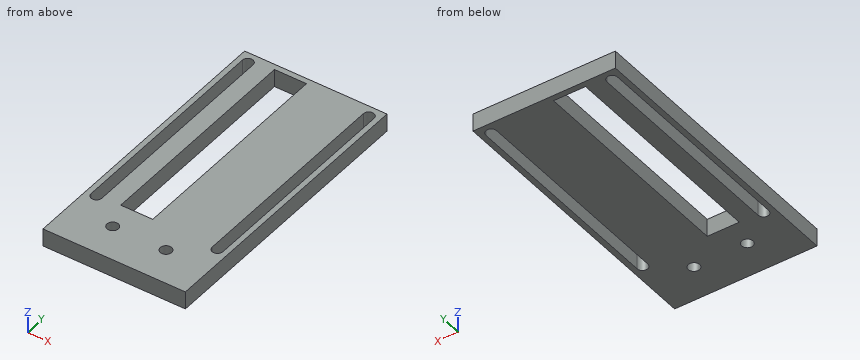
from build123d import *

# Parameters (mm, degrees)
SKETCH1_W           = 40
SKETCH1_H           = 20
SKETCH1_R           = 1.6
BOSS_EXTRUDE1_DEPTH = 5
SKETCH3_W           = 40
SKETCH3_H           = 5
BOSS_EXTRUDE3_DEPTH = 60
CUT_EXTRUDE1_DEPTH  = 73.972597597
SKETCH5_W           = 9
SKETCH5_H           = 60.997272609
CUT_EXTRUDE2_DEPTH  = 73.972597597


with BuildPart() as part:
    # Sketch1 → Boss-Extrude1 (new body)
    with BuildSketch(Plane.XY):
        Rectangle(SKETCH1_W, SKETCH1_H)
        with Locations((-7.5, 0)):
            Circle(SKETCH1_R, mode=Mode.SUBTRACT)
        with Locations((7.5, 0)):
            Circle(SKETCH1_R, mode=Mode.SUBTRACT)
    extrude(amount=BOSS_EXTRUDE1_DEPTH)

    # Sketch3 → Boss-Extrude3 (add)
    with BuildSketch(Plane(origin=(0, 10, 0), x_dir=(1, 0, 0), z_dir=(0, 1, 0))):
        with Locations((0, -2.5)):
            Rectangle(SKETCH3_W, SKETCH3_H)
    extrude(amount=BOSS_EXTRUDE3_DEPTH)

    # Sketch4 → Cut-Extrude1 (cut, through all)
    with BuildSketch(Plane(origin=(0, 0, 0), x_dir=(-1, 0, 0), z_dir=(0, 0, -1))):
        with BuildLine():
            Line((-15.5, 67), (-15.5, 7))
            ThreePointArc((-15.5, 7), (-17, 5.5), (-18.5, 7))
            Line((-18.5, 7), (-18.5, 67))
            ThreePointArc((-18.5, 67), (-17, 68.5), (-15.5, 67))
        make_face()
        with BuildLine():
            Line((18.5, 67), (18.5, 7))
            ThreePointArc((18.5, 7), (17, 5.5), (15.5, 7))
            Line((15.5, 7), (15.5, 67))
            ThreePointArc((15.5, 67), (17, 68.5), (18.5, 67))
        make_face()
    extrude(amount=-CUT_EXTRUDE1_DEPTH, mode=Mode.SUBTRACT)

    # Sketch5 → Cut-Extrude2 (cut, through all)
    with BuildSketch(Plane(origin=(0, 0, 0), x_dir=(-1, 0, 0), z_dir=(0, 0, -1))):
        with Locations((6, 37.926958335)):
            Rectangle(SKETCH5_W, SKETCH5_H)
    extrude(amount=-CUT_EXTRUDE2_DEPTH, mode=Mode.SUBTRACT)


solid = part.part
Model file for the job. Use its own axes, mm. Give positions to 0.01 mm unless a question says otherwise; leave off trailing zeros. Write each loop counter-clockwise with the first axis right and the second up, starting at its lowest first coordinate (ties: lowest second). Pieces come first, ordered by that corner, then holes. Notation, with made-up numbers: M 83,32 L 130,32 A19 cw 130,66 Z; hole C 83.5,54 d1. An arc over 180 degrees is marked long. One line per item, written item: value. Start each with the question number.
Q1. Saw through at A-A, the plane x = -7.5. Write the cut outline in (y, z), plus the area to 3 significant figures.
Q2. Probe probe 1 along X at (y, z) = (35, 1); probe 2 along Y at (x, z) = (-7.5, 3.75); probe 3 along Y at (x, z) = (7.5, 2.3). List the from-to ranges inside material, lowest first. Write a range as [from, to].
Q3. Saw through at C-C, the plane z = 0.9. Write the cut outline in (x, y), plus the area to 3 significant figures.
Q4. Saw through at D-D, the plane x = -17. Write the cut outline in (y, z), plus the area to 3 significant figures.
Q5. Drop a flat-ended pin along its axis: pin 1 Ø12 at (x, y) = (-11, 6) entering from -Z. Give the stop position or say it passes through.
Q6. Saw through at B-B, the plane y = 39.5. Write the cut outline in (x, z), plus the area to 3 significant figures.
Output values:
1. outline: M -10,0 L -1.6,0 L -1.6,5 L -10,5 Z; M 1.6,0 L 7.43,0 L 7.43,5 L 1.6,5 Z; M 68.43,0 L 70,0 L 70,5 L 68.43,5 Z
1. area: 79.0 mm²
2. probe 1: x = [-20, -18.5], [-15.5, -10.5], [-1.5, 15.5], [18.5, 20]
2. probe 2: y = [-10, -1.6], [1.6, 7.43], [68.43, 70]
2. probe 3: y = [-10, -1.6], [1.6, 70]
3. outline: M -20,-10 L 20,-10 L 20,70 L -20,70 Z; hole M -18.5,7 A1.5 ccw -15.5,7 L -15.5,67 A1.5 ccw -18.5,67 Z; hole M -10.5,7.43 L -1.5,7.43 L -1.5,68.43 L -10.5,68.43 Z; hole C -7.5,0 d3.2; hole C 7.5,0 d3.2; hole M 15.5,7 A1.5 ccw 18.5,7 L 18.5,67 A1.5 ccw 15.5,67 Z
3. area: 2,260 mm²
4. outline: M -10,0 L 5.5,0 L 5.5,5 L -10,5 Z; M 68.5,0 L 70,0 L 70,5 L 68.5,5 Z
4. area: 85.0 mm²
5. pin 1: stops at z = 0
6. outline: M -20,0 L -18.5,0 L -18.5,5 L -20,5 Z; M -15.5,0 L -10.5,0 L -10.5,5 L -15.5,5 Z; M -1.5,0 L 15.5,0 L 15.5,5 L -1.5,5 Z; M 18.5,0 L 20,0 L 20,5 L 18.5,5 Z
6. area: 125 mm²
